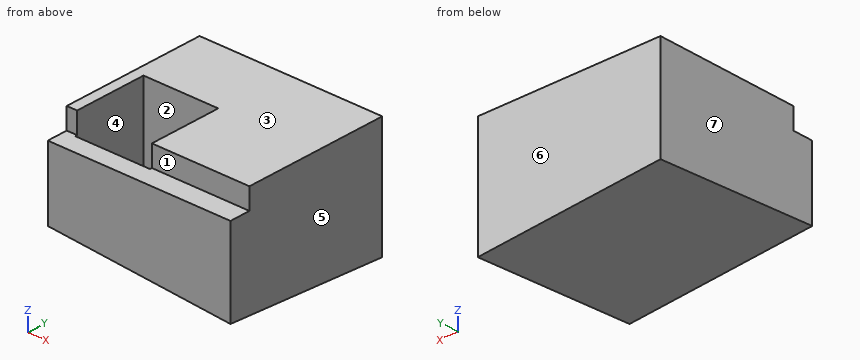
```python
from build123d import *

# Parameters (mm, degrees)
BOX003_W               = 24
BOX003_H               = 23
BOX003_DEPTH           = 10
BOX003_ROLL_ANGLE      = -3.799965
BOX003_PITCH_ANGLE     = 4.646714
BOX003_PLACEMENT_ANGLE = -0.15423
BOX002_W               = 22
BOX002_H               = 2.5
BOX002_DEPTH           = 2.5
BOX001_W               = 9
BOX001_H               = 9
BOX001_DEPTH           = 11
BOX_W                  = 22
BOX_H                  = 20
BOX_DEPTH              = 15


with BuildPart() as cube003:
    # Box003 → Box003 (new body)
    with BuildSketch(Plane.XY):
        with Locations((12, 11.5)):
            Rectangle(BOX003_W, BOX003_H)
    extrude(amount=BOX003_DEPTH)


with BuildPart() as cube003_1:
    # Box003 roll: moved
    add(cube003.part.rotate(Axis((0, 0, 0), (1, 0, 0)), BOX003_ROLL_ANGLE))


with BuildPart() as cube003_2:
    # Box003 pitch: moved
    add(cube003_1.part.rotate(Axis((0, 0, 0), (0, 1, 0)), BOX003_PITCH_ANGLE))


with BuildPart() as cube003_3:
    # Box003 placement: moved
    add(cube003_2.part.moved(Location((-1, -2, -6))).rotate(Axis((-1, -2, -6), (0, 0, 1)), BOX003_PLACEMENT_ANGLE))


with BuildPart() as cube002:
    # Box002 → Box002 (new body)
    with BuildSketch(Plane.XY.offset(12.5)):
        with Locations((11, 1.25)):
            Rectangle(BOX002_W, BOX002_H)
    extrude(amount=BOX002_DEPTH)


with BuildPart() as cube001:
    # Box001 → Box001 (new body)
    with BuildSketch(Plane(origin=(1.25, 2.25, 4), x_dir=(1, 0, 0), z_dir=(0, 0, 1))):
        with Locations((4.5, 4.5)):
            Rectangle(BOX001_W, BOX001_H)
    extrude(amount=BOX001_DEPTH)


with BuildPart() as cut002:
    # Box → Box (new body)
    with BuildSketch(Plane.XY):
        with Locations((11, 10)):
            Rectangle(BOX_W, BOX_H)
    extrude(amount=BOX_DEPTH)

    # Cut: cut Cube001
    add(cube001.part, mode=Mode.SUBTRACT)

    # Cut001: cut Cube002
    add(cube002.part, mode=Mode.SUBTRACT)

    # Cut002: cut Cube003
    add(cube003_3.part, mode=Mode.SUBTRACT)


solid = cut002.part
```
Geometry check sheet. Reference: the model listing, model coordinates, mm. Face numbers are marked on the shaded views. A direction names the side the tool comes from. Round coordinates to 2 decimals unless told otherwise and drop trailing zeros. Loops run counter-clockwise (first coordinate to the right, second up) from the corner with the lowest first, then second, coordinate; pieces in that order, holes last. Notation, with made-up numbers: (-21, 83.25) -> (28, 83.25) arc R16 ccw to (28, 97.25) -> close; hole circle Ø2 at (5, -4). An arc over 180 degrees is marked (long way). Use a Markdown table: item, result.
(1) Go/stop test with flat-tipped pins: P1, Ø1, axis at x = 4.5, y = 14.5, coming from the -Z side; P2, Ø1.2, axis at x = 14.5, y = 1, coming from the +Z side; P3, Ø3, axis at x = 13.5, y = 10, coming from the -Z side. Record where each tip stops, or that it passes through.
Calculated:
| item | result |
|---|---|
| P1 | z = 2.46 |
| P2 | z = 12.5 |
| P3 | z = 1.92 |
(2) Sectioned sample at B-B (z = 14.25). Enter the section's corners in (x, y), then the cut area to 3 significant figures.
Calculated:
| item | result |
|---|---|
| outline | (0, 2.5) -> (1.25, 2.5) -> (1.25, 11.25) -> (10.25, 11.25) -> (10.25, 2.5) -> (22, 2.5) -> (22, 20) -> (0, 20) -> close |
| area | 306 mm² |
(3) Sectioned sample at C-C (x = 2.5). Enter the section's corners in (y, z), then the cut area to 3 significant figures.
Calculated:
| item | result |
|---|---|
| outline | (0, 3.64) -> (20, 2.31) -> (20, 15) -> (11.25, 15) -> (11.25, 4) -> (2.25, 4) -> (2.25, 12.5) -> (0, 12.5) -> close |
| area | 136 mm² |
(4) Mould release check, pull along X, two halves, no side actions. Record for the marked faces 4, 5, 6 and 7: released by +X, released by -X, zero draft, split by the parting line, or undercut.
Calculated:
| item | result |
|---|---|
| face 4 | undercut |
| face 5 | released by +X |
| face 6 | zero draft |
| face 7 | released by -X |
(5) Set-up check for the marked faces 1, 2 and 3: record each of +Z, -Z, +X, -X, +Y, -Y from which the full face is reachable in a straight line by a thin tool's end or side.
Calculated:
| item | result |
|---|---|
| face 1 | +Z, +X, -X, -Y |
| face 2 | +Z |
| face 3 | +Z, +X, -X, +Y, -Y |
(6) Sectioned sample at A-A (z = 8.25). Enter the section's corners in (x, y), then the cut area to 3 significant figures.
Calculated:
| item | result |
|---|---|
| outline | (0, 0) -> (22, 0) -> (22, 20) -> (0, 20) -> close; hole (1.25, 2.25) -> (10.25, 2.25) -> (10.25, 11.25) -> (1.25, 11.25) -> close |
| area | 359 mm² |
(7) Scan lines: probe 1 along X at (y, z) = (8.5, 13.25); probe 2 along Y at (x, z) = (5.75, 12.25); probe 3 along Z at (x, y) = (16.5, 8.25). Record each from-to range of solid material in increasing order.
Calculated:
| item | result |
|---|---|
| probe 1 | 0 to 1.25, 10.25 to 22 |
| probe 2 | 0 to 2.25, 11.25 to 20 |
| probe 3 | 1.95 to 15 |
(8) Sectioned sample at D-D (y = 17.75). Enter the section's corners in (x, z).
Calculated:
| item | result |
|---|---|
| outline | (0, 2.66) -> (22, 0.87) -> (22, 15) -> (0, 15) -> close |
